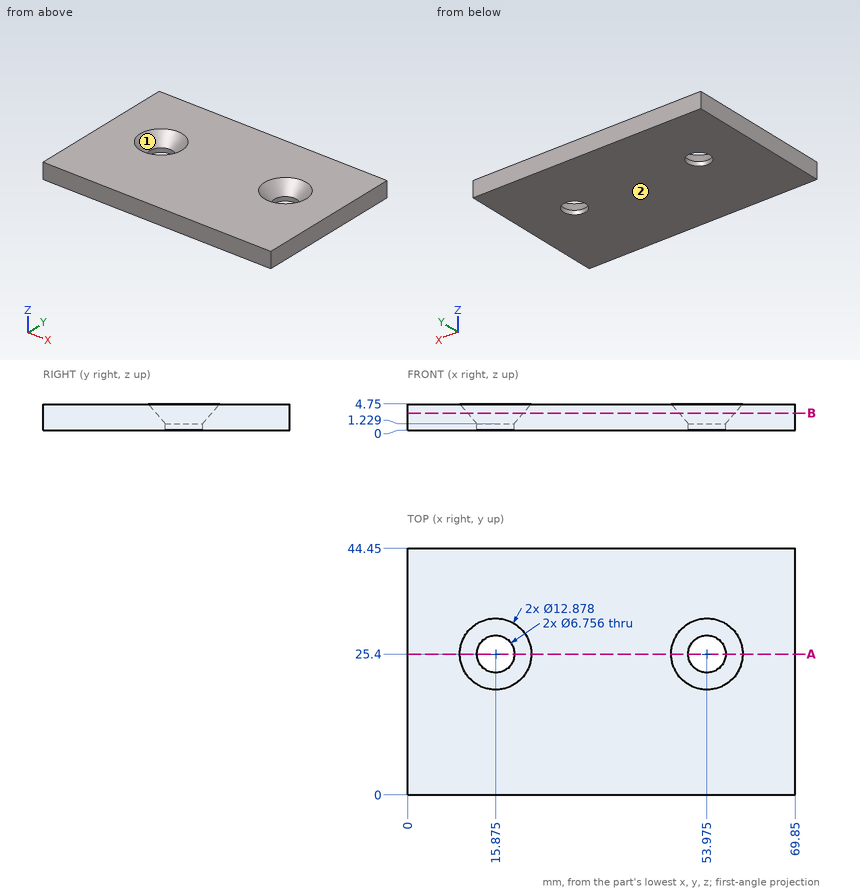
Could you check a few things on this drawing? It's one solid part, dimensions in mm from its lowest x, y, z. Give positions to 0.01 mm unless a question says otherwise; leave off trailing zeros. Order: outer loops, then holes, each group sorted by start corner. A loop starts at its lowest first (then second) coordinate and runs counter-clockwise, first axis right, second up. Notation, with made-up numbers: (79, 54) -> (137, 54) arc R21 ccw to (137, 71) -> close; hole circle Ø5 at (2.25, 44.25). An arc over 180 degrees is marked (long way). Answer in a Markdown table with one row per item. Add a question column.
Item 1: We'd pull the mould along Y, two halves only. Please class the marked faces 1 and 2: pulls with the +Y half, pulls with the -Y half, needs draft (parallel to the pull), parting line crosses it, or undercut.
Item 2: Please list where these lines run through material, in increasing order: probe 1 along X at (y, z) = (25.4, 0.45); probe 2 along Y at (x, z) = (56, 4.05); probe 3 along Y at (x, z) = (58, 4.4).
Item 3: Imagine slicing it at B-B (z = 3.1). Count the separate pieces of the cut face and the enclosed holes in it, and give its area (3 significant figures).
Item 4: I'm going to push flat-ended pins straight in: P1, Ø4, axis at x = 53.975, y = 25.4, coming from the +Z side; P2, Ø3, axis at x = 22, y = 24, coming from the +Z side; P3, Ø8, axis at x = 15.875, y = 25.4, coming from the +Z side (1 decimal). Where does each tip first touch, or does it pass through?
Item 5: Imagine slicing it at A-A (y = 25.4). List the corners of the cut face in (x, z) for me.
Result:
| question | item | result |
|---|---|---|
| 1 | face 1 | undercut |
| 1 | face 2 | needs draft |
| 2 | probe 1 | 0 to 12.5, 19.25 to 50.6, 57.35 to 69.85 |
| 2 | probe 2 | 0 to 19.93, 30.87 to 44.45 |
| 2 | probe 3 | 0 to 20.77, 30.03 to 44.45 |
| 3 | separate pieces | 1 |
| 3 | enclosed holes | 2 |
| 3 | area | 2,950 mm2 |
| 4 | P1 | through |
| 4 | P2 | z = 4.75 |
| 4 | P3 | z = 1.9 |
| 5 | outline | (0, 0) -> (12.5, 0) -> (12.5, 1.23) -> (9.44, 4.75) -> (0, 4.75) -> close; (19.25, 0) -> (50.6, 0) -> (50.6, 1.23) -> (47.54, 4.75) -> (22.31, 4.75) -> (19.25, 1.23) -> close; (57.35, 0) -> (69.85, 0) -> (69.85, 4.75) -> (60.41, 4.75) -> (57.35, 1.23) -> close |
